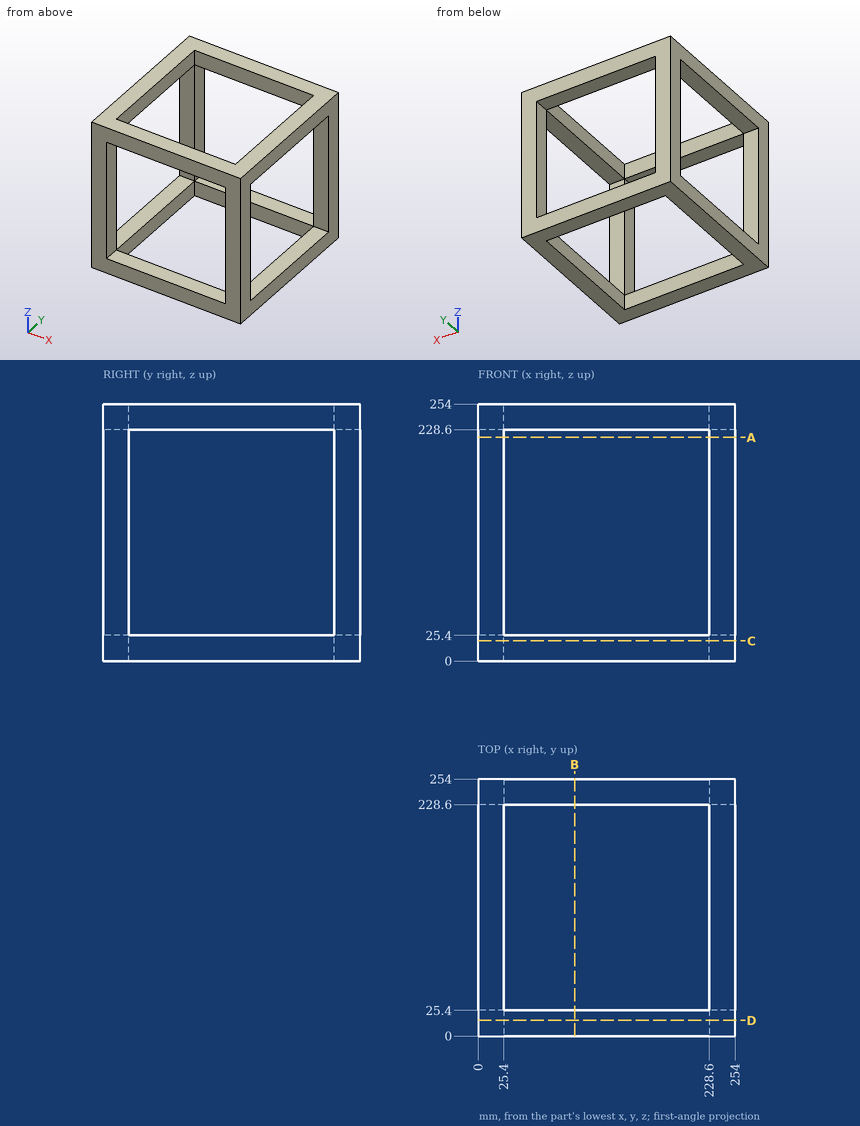
Geometry: see drawing. Coordinates: mm, zero at the bounding-box minimum. Give positions to 0.01 mm unless a question says otherwise; leave off trailing zeros. Order: outer loops, then holes, each group sorted by start corner. A loop starts at its lowest first (then second) coordinate and runs counter-clockwise, first axis right, second up.
Q1. Section C-C on z = 20. Output: boundary loops of the cut face in (x, y), and give its area (3 significant figures).
Checked values:
outline: (0, 0) - (254, 0) - (254, 254) - (0, 254) - close; hole (25.4, 25.4) - (228.6, 25.4) - (228.6, 228.6) - (25.4, 228.6) - close
area: 23,200 mm2
Q2. Ray query, probe 1 along Z at (x, y) = (195, 234). Return the intervals inside material, ascending.
Checked values:
probe 1: z = 0 to 25.4, 228.6 to 254
Q3. Section A-A on z = 221. Output: boundary loops of the cut face in (x, y).
Checked values:
outline: (0, 0) - (25.4, 0) - (25.4, 25.4) - (0, 25.4) - close; (0, 228.6) - (25.4, 228.6) - (25.4, 254) - (0, 254) - close; (228.6, 0) - (254, 0) - (254, 25.4) - (228.6, 25.4) - close; (228.6, 228.6) - (254, 228.6) - (254, 254) - (228.6, 254) - close
